The listing builds one solid part. Answer for the finished solid, in the listing's coordinates (mm). Give positions to 0.01 mm unless a question says otherwise; leave off trailing zeros. Order: outer loops, then holes, each group sorted by start corner. A loop starts at its lowest first (then second) coordinate and runs counter-clockwise, first axis right, second up.
```python
from build123d import *
from build123d.topology import SkipClean

# Parameters (mm, degrees)
SALIENTE_EXTRUIR1_START = 0.2
CROQUIS1_R              = 1.75
SALIENTE_EXTRUIR1_DEPTH = 3.6
CROQUIS2_R              = 3.40408827
CROQUIS2_R_2            = 1.75
SALIENTE_EXTRUIR2_DEPTH = 6.2


with BuildPart() as part:
    # Croquis1 → Saliente-Extruir1 (new body)
    with BuildSketch(Plane.XY.offset(SALIENTE_EXTRUIR1_START)):
        with BuildLine():
            Line((-80.917805582, 11.650275301), (-67.150813208, -4.628100839))
            ThreePointArc((-67.150813208, -4.628100839), (-67.552307173, -9.425900411), (-72.350029665, -9.023486412))
            Line((-72.350029665, -9.023486412), (-86.110777841, 7.260168535))
            ThreePointArc((-86.110777841, 7.260168535), (-85.708924205, 12.051210184), (-80.917805582, 11.650275301))
        make_face()
        with Locations((-69.75, -6.826292135)):
            Circle(CROQUIS1_R, mode=Mode.SUBTRACT)
        with Locations((-83.513870781, 9.454724007)):
            Circle(CROQUIS1_R, mode=Mode.SUBTRACT)
    saliente_extruir1 = extrude(amount=SALIENTE_EXTRUIR1_DEPTH)

    # Croquis2 → Saliente-Extruir2 (add)
    with SkipClean():  # the faces are left unmerged after this step: merging them gives an invalid solid
        with BuildSketch(Plane.XY.offset(3.8)):
            with Locations(Location((-69.75, -6.826292135, 0), (0, 0, 220.199985321))):
                Circle(CROQUIS2_R)
            with Locations(Location((-69.75, -6.826292135, 0), (0, 0, 90))):
                Circle(CROQUIS2_R_2, mode=Mode.SUBTRACT)
        saliente_extruir2 = extrude(amount=SALIENTE_EXTRUIR2_DEPTH)

    # Simetría1: Saliente-Extruir2 across plane
    with SkipClean():  # the faces are left unmerged after this step: merging them gives an invalid solid
        add(saliente_extruir2.mirror(Plane(origin=(0, 0, 10), x_dir=(1, 0, 0), z_dir=(0, 0, -1))))

    # Simetría4: Saliente-Extruir1 across plane
    with SkipClean():  # the faces are left unmerged after this step: merging them gives an invalid solid
        add(saliente_extruir1.mirror(Plane(origin=(0, 0, 10), x_dir=(1, 0, 0), z_dir=(0, 0, -1))))


solid = part.part
```
1) Find section D-D (z = 17.75). Write down the section's boundary in (x, y), then the cut area to 3 significant figures.
Geometry says:
outline: (-86.11, 7.26) - (-72.35, -9.02) arc R3.4 ccw to (-67.15, -4.63) - (-80.92, 11.65) arc R3.4 ccw to start; hole circle Ø3.5 at (-83.51, 9.45); hole circle Ø3.5 at (-69.75, -6.83)
area: 162 mm2
2) Find section C-C (y = 10.75). Write down the section's boundary in (x, z), then the cut area to 3 significant figures.
Geometry says:
outline: (-86.66, 0.2) - (-84.69, 0.2) - (-84.69, 3.8) - (-86.66, 3.8) - close; (-86.66, 16.2) - (-84.69, 16.2) - (-84.69, 19.8) - (-86.66, 19.8) - close; (-82.34, 0.2) - (-80.16, 0.2) - (-80.16, 3.8) - (-82.34, 3.8) - close; (-82.34, 16.2) - (-80.16, 16.2) - (-80.16, 19.8) - (-82.34, 19.8) - close
area: 29.9 mm2
3) For a pull along Y with two mould halves and no side action, classify faces 1 (the flat face through (-79.13, -1, 18.03)), 2 (the cylindrical face through (-81.845, 9.98, 1.975)), 3 (the flat face through (-76, 1, 0.2)) as +Y half, -Y half, draft (parallel to the pull), parting line (faces both ways), or undercut.
Geometry says:
face 1: -Y half
face 2: undercut
face 3: draft
4) Given P1, Ø2, axis at x = -83.51, y = 9.45, coming from the +Z side; P2, Ø4, axis at x = -69.75, y = -6.83, coming from the -Z side; P3, Ø8, axis at y = 0.5, z = 4.5, coming from the +X side; P4, Ø5, axis at y = -1, z = 17.5, coming from the -X side, each flat-ended and moving along its own axis, determine where each tip first touches the part or whether it passes through.
Geometry says:
P1: passes through
P2: stops at z = 0.2
P3: stops at x = -68.16
P4: stops at x = -81.24
5) Find section B-B (y = 3.25). Write down the section's boundary in (x, z).
Geometry says:
outline: (-82.72, 0.2) - (-73.81, 0.2) - (-73.81, 3.8) - (-82.72, 3.8) - close; (-82.72, 16.2) - (-73.81, 16.2) - (-73.81, 19.8) - (-82.72, 19.8) - close
6) Find section A-A (x = -75.25). Write down the section's boundary in (y, z).
Geometry says:
outline: (-5.59, 0.2) - (4.95, 0.2) - (4.95, 3.8) - (-5.59, 3.8) - close; (-5.59, 16.2) - (4.95, 16.2) - (4.95, 19.8) - (-5.59, 19.8) - close
7) Straight lines are drawn through the part: probe 1 along Z at (x, y) = (-77.25, 6); probe 2 along Y at (x, z) = (-69.75, 7); probe 3 along Y at (x, z) = (-69.75, 18.5). For each, find the intervals that lie inside material, in ascending order.
Geometry says:
probe 1: z = 0.2 to 3.8, 16.2 to 19.8
probe 2: y = -10.23 to -8.58, -5.08 to -3.42
probe 3: y = -10.23 to -8.58, -5.08 to -1.55
